For this review, take the finished solid that the model builds, in its own axes (mm). Face numbers are marked on the shaded views. A direction names the side the tool comes from. Coordinates: 2 decimals unless noted, no trailing zeros. Loops run counter-clockwise (first coordinate to the right, second up) from the corner with the lowest first, then second, coordinate; pieces in that order, holes last. Notation, with made-up numbers: M -16,-26 L 38,-26 A21 ccw 38,-16 Z; hole C 37,61.5 d7. An arc over 180 degrees is marked long. Answer as a JSON object with one key per item and string values. Group by question number.
Item 1: Insertion check: pin 1 (1.5 mm diameter, centred on y = 5, z = 3, fed in from +X); pin 2 (0.5 mm diameter, centred on x = 3.5, y = -2, fed in from -Z); pin 3 (1.8 mm diameter, centred on x = -0.5, z = 3, fed in from -Y); pin 4 (1.5 mm diameter, centred on x = -1, z = 1.5, fed in from -Y). Each pin has a flat end and moves straight along its axis. Give the tip position at first contact, or say it passes through.
Item 2: Add section D-D (y = -1.5). State the section outline as (x, z) points, then the cut area to 3 significant figures.
Item 3: Tool access review of the marked faces 5, 6 and 7: name each direction out of +Z, -Z, +X, -X, +Y, -Y from which nothing blocks a thin tool from reaching the whole face with its end or side.
Item 4: Wall thickness on L1, parallel to Z at x = 0, y = -8.35; L2, parallel to X at y = -8.3, z = 2.5; L3, parallel to Y at x = 0.25, z = 2.1: over which ranges is each line inside the solid? List them lowest first. Write a range as from..to.
Item 5: Add section B-B (x = 2). State the section outline as (y, z) points.
Item 6: Mouldability with a two-part tool opening along Y and no side actions: class the marked faces 1, 2, 3 and 4 as +Y half, -Y half, draft (parallel to the pull), parting line (faces both ways), or undercut.
Item 7: Add section A-A (y = 3.75). State the section outline as (x, z) points, then the cut area to 3 significant figures.
Item 8: Add section C-C (z = 2.5). State the section outline as (x, y) points (3 decimals), then the cut area to 3 significant figures.
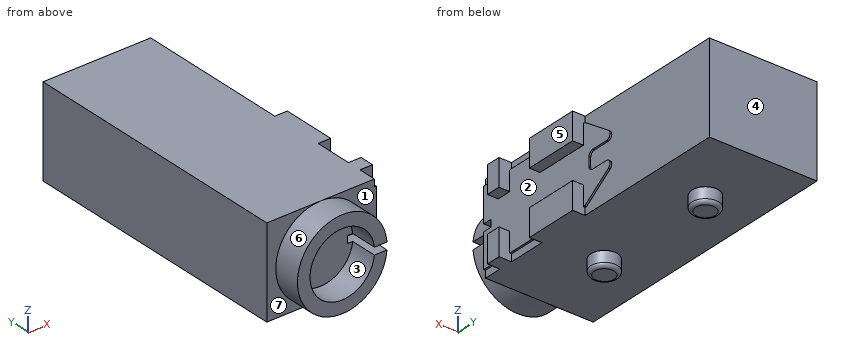
Autodesk Inventor part; units mm, degrees
ref_plane "YZ Plane" through (0, 0, 0) normal (1, 0, 0) x (0, 1, 0)
ref_plane "XZ Plane" through (0, 0, 0) normal (0, 1, 0) x (-1, 0, 0)
ref_plane "XY Plane" through (0, 0, 0) normal (0, 0, 1) x (1, 0, 0)
sketch "Sketch1" plane through (0, 0, 0) normal (0, 0, 1) x (1, 0, 0)
  line L0 (3, -7.75) -> (-3, -7.75)
  line L1 (-3, -7.75) -> (-3, 7.75)
  line L2 (-3, 7.75) -> (3, 7.75)
  line L3 (3, 7.75) -> (3, -7.75)
  line L4 (3, -7.75) -> (-3, 7.75) construction
  line L5 (-3, -7.75) -> (3, 7.75) construction
  point P0 (0, 0)
  dimension "d0" = 6
  dimension "d1" = 15.5
extrude "Extrusion1" add sketch "Sketch1" along normal blind 5
sketch "Sketch2" plane through (-3, -7.75, 0) normal (0, -1, 0) x (1, 0, 0)
  line L0 (6, 0) -> (0, 0)
  line L1 (6, 0) -> (6, 5)
  line L2 (0, 5) -> (6, 5)
  line L3 (0, 0) -> (0, 5)
  line L4 (6, 0) -> (0, 0)
  line L5 (0, 0) -> (6, 5)
  circle A0 centre (3, 2.5) radius 2.5
  circle A1 centre (3, 2.5) radius 1.8
  point P0 (3, 0)
  dimension "d4" = 5
  dimension "d5" = 3.6
extrude "Extrusion2" add sketch "Sketch2" along normal blind 1.5 contours A0 L5 A1 | A0 L5 A1
sketch "Sketch3" plane through (0, 0, 0) normal (0, 0, -1) x (-1, 0, 0)
  line L0 (-3, -7.75) -> (0, -7.75)
  line L1 (0, -7.75) -> (3, -7.75)
  line L2 (3, -7.75) -> (3, 7.75)
  line L3 (3, 7.75) -> (-3, 7.75)
  line L4 (-3, 7.75) -> (-3, -7.75)
  circle A0 centre (0, -3.25) radius 0.75
  circle A1 centre (0, 3.75) radius 0.75
  point P0 (0, 0)
  dimension "d8" = 1.5
  dimension "d9" = 1.5
  dimension "d10" = 4.5
  dimension "d11" = 7
extrude "Extrusion3" add sketch "Sketch3" along normal blind 0.8 contours A0 | A1
fillet "Fillet1" radius 0.2 2 edges at (0.75, -3.25, -0.8) (0.75, 3.75, -0.8)
sketch "Sketch4" plane through (3, -7.75, 0) normal (1, 0, 0) x (0, 0, -1)
  line L0 (0, 15.5) -> (0, 0)
  line L1 (0, 15.5) -> (-5, 15.5)
  line L2 (-5, 0) -> (-5, 15.5)
  line L3 (0, 0) -> (-5, 0)
  line L4 (-5, 15.5) -> (-5, 0)
  line L5 (-5, 1) -> (-3.5, 1)
  line L6 (-3.5, 1) -> (-3.5, 1.8)
  line L7 (-3.5, 1.8) -> (-5, 1.8)
  line L8 (-5, 1.8) -> (-5, 1)
  line L9 (0, 1) -> (-1.5, 1)
  line L10 (-1.5, 1) -> (-1.5, 1.8)
  line L11 (-1.5, 1.8) -> (0, 1.8)
  line L12 (0, 1.8) -> (0, 1)
  line L13 (-5, 3.9) -> (-3.5, 3.9)
  line L14 (-3.5, 3.9) -> (-3.5, 6.9)
  line L15 (-3.5, 6.9) -> (-5, 6.9)
  line L16 (-5, 6.9) -> (-5, 3.9)
  line L17 (0, 3.9) -> (-1.5, 3.9)
  line L18 (-1.5, 3.9) -> (-1.5, 6.9)
  line L19 (-1.5, 6.9) -> (0, 6.9)
  line L20 (0, 6.9) -> (0, 3.9)
  point P0 (0, 7.75)
  dimension "d15" = 1
  dimension "d16" = 0.8
  dimension "d17" = 1.5
  dimension "d18" = 1.5
  dimension "d19" = 1.5
  dimension "d20" = 1.5
  dimension "d21" = 3.9
  dimension "d22" = 3
extrude "Extrusion4" add sketch "Sketch4" along normal blind 0.7 contours L0 L17 L18 L19 | L15 L14 L13 L2 | L0 L9 L10 L11 | L7 L6 L5 L2
sketch "Sketch5" plane through (3, 7.75, 5) normal (1, 0, 0) x (0, 0, -1)
  line L0 (3.5, -8.6) -> (5, -8.6)
  line L1 (5, 0) -> (5, -8.6)
  line L2 (5, 0) -> (0, 0)
  line L3 (0, -8.6) -> (0, 0)
  line L4 (0, -8.6) -> (1.5, -8.6)
  line L5 (1.5, -8.6) -> (1.5, -11.6)
  line L6 (1.5, -11.6) -> (0, -11.6)
  line L7 (0, -13.7) -> (0, -11.6)
  line L8 (0, -13.7) -> (1.5, -13.7)
  line L9 (1.5, -13.7) -> (1.5, -14.5)
  line L10 (1.5, -14.5) -> (0, -14.5)
  line L11 (0, -15.5) -> (0, -14.5)
  line L12 (5, -15.5) -> (0, -15.5)
  line L13 (5, -14.5) -> (5, -15.5)
  line L14 (5, -14.5) -> (3.5, -14.5)
  line L15 (3.5, -14.5) -> (3.5, -13.7)
  line L16 (3.5, -13.7) -> (5, -13.7)
  line L17 (5, -11.6) -> (5, -13.7)
  line L18 (5, -11.6) -> (3.5, -11.6)
  line L19 (3.5, -11.6) -> (3.5, -8.6)
  line L20 (0.4, -15.5) -> (0.4, -8.5)
  line L21 (0, -8.6) -> (1.5, -8.6)
  line L22 (0.4, -8.5) -> (1.5452, -6.8645)
  line L23 (2, -7.0079) -> (2, -7.965)
  line L24 (2.25, -8.215) -> (2.75, -8.215)
  line L25 (3, -7.965) -> (3, -7.0079)
  line L26 (3.4548, -6.8645) -> (4.6, -8.5)
  line L27 (4.6, -8.5) -> (4.6, -15.5)
  line L28 (5, -15.5) -> (0, -15.5)
  line L29 (2.5, -15.5) -> (2.5, 0)
  line L30 (5, 0) -> (0, 0)
  arc A0 (3.4548, -6.8645) -> (3, -7.0079) centre (3.25, -7.0079) ccw
  arc A1 (2, -7.0079) -> (1.5452, -6.8645) centre (1.75, -7.0079) ccw
  arc A2 (2, -7.965) -> (2.25, -8.215) centre (2.25, -7.965) ccw
  arc A3 (2.75, -8.215) -> (3, -7.965) centre (2.75, -7.965) ccw
  point P0 (5, -7.75)
  point P1 (2, -8.215)
  point P2 (3, -8.215)
  point P3 (3, -6.215)
  point P4 (2.5, -8.215)
  dimension "d25" = 0.4
  dimension "d26" = 0.4
  dimension "d27" = 145
  dimension "d28" = 145
  dimension "d29" = 1
  dimension "d30" = 7
  dimension "d31" = 7
  dimension "d32" = 2
  dimension "d33" = 0.25
extrude "Extrusion5" add sketch "Sketch5" along normal blind 0.1 contours L19 L18 L27 L16 L15 L14 L12 L29 L24 A3 L25 A0 L26 L0 | L0 L27 L18 L19 | L27 L14 L15 L16 | L29 L12 L20 L10 L9 L8 L6 L5 L4 L22 A1 L23 A2 L24 | L4 L5 L6 L20 | L20 L8 L9 L10
sketch "Sketch6" plane through (0, -9.25, 2.5) normal (0, -1, 0) x (1, 0, 0)
  circle A0 centre (0, 0) radius 1.8
  circle A1 centre (0, 0) radius 2.5
  line L0 (1.5, -0.2) -> (3.5, -0.2)
  line L1 (3.5, -0.2) -> (3.5, 0.2)
  line L2 (3.5, 0.2) -> (1.5, 0.2)
  line L3 (1.5, 0.2) -> (1.5, -0.2)
  line L4 (1.5, -0.2) -> (3.5, 0.2) construction
  line L5 (3.5, -0.2) -> (1.5, 0.2) construction
  point P0 (0, -2.5)
  point P1 (2.5, 0)
  dimension "d36" = 2
  dimension "d37" = 0.4
extrude "Extrusion6" cut sketch "Sketch6" against normal blind 2 contours A0 L0 L3 L2 | A0 L2 A1 L0 | L2 L1 L0 A1 picked at (1.6, 0) picked at (2.0301, 0.1112)
equation "\"d18\" = d17"
equation "\"d19\" = d17"
equation "\"d20\" = d18"
equation "\"d26\" = d25"
equation "\"d31\" = d30"
properties part number "SJ-4351X-SMT" material "ABS Plastic"
From the geometry:
{
 "1": {"pin 1": "stops at x = 3", "pin 2": "stops at z = 0", "pin 3": "stops at y = -7.75", "pin 4": "stops at y = -9.25"},
 "2": {"outline": "M -3,0 L 3.7,0 L 3.7,1.5 L 3.1,1.5 L 3.1,3.5 L 3.7,3.5 L 3.7,5 L -3,5 Z", "area": "32.3 mm²"},
 "3": {"face 5": "+Z, -Z, +X, +Y, -Y", "face 6": "-Y", "face 7": "-X, -Y"},
 "4": {"L1": "z = 0..0.7, 4.3..5", "L2": "x = -2.5..-1.8", "L3": "y = -7.75..7.75"},
 "5": {"outline": "M -9.25,1 L -7.75,1 L -7.75,0 L 7.75,0 L 7.75,5 L -7.75,5 L -7.75,4 L -9.25,4 L -9.25,2.7 L -7.25,2.7 L -7.25,2.3 L -9.25,2.3 Z"},
 "6": {"face 1": "-Y half", "face 2": "undercut", "face 3": "draft", "face 4": "+Y half"},
 "7": {"outline": "M -3,0 L -0.75,0 L -0.75,-0.6 A0.2 ccw -0.55,-0.8 L 0.55,-0.8 A0.2 ccw 0.75,-0.6 L 0.75,0 L 3,0 L 3,5 L -3,5 Z", "area": "31.2 mm²"},
 "8": {"outline": "M -3,-7.75 L -2.5,-7.75 L -2.5,-9.25 L -1.8,-9.25 L -1.8,-7.75 L 1.5,-7.75 L 1.5,-7.25 L 3.1,-7.25 L 3.1,-0.465 L 3,-0.465 L 3,7.75 L -3,7.75 Z", "area": "94.0 mm²"}
}
